Design review of the part built by this model. Coordinates are the model's own, in mm. Face numbers are marked on the shaded views. A direction names the side the tool comes from. Round coordinates to 2 decimals unless told otherwise and drop trailing zeros. Order: outer loops, then holes, each group sorted by start corner. A loop starts at its lowest first (then second) coordinate and runs counter-clockwise, first axis right, second up. Notation, with made-up numbers: (28.5, -1) - (52.5, -1) arc R19 ccw to (52.5, 30) - close; hole circle Ø5 at (65.5, -21). An arc over 180 degrees is marked (long way). Write item = value, one per line.
Autodesk Inventor part; units mm, degrees
ref_plane "XZ Plane" through (0, 0, 0) normal (0, 1, 0) x (-1, 0, 0)
sketch "Sketch1" plane through (0, 0, 0) normal (0, 1, 0) x (-1, 0, 0)
  line L0 (60.4, 85.9) -> (-60.4, 85.9)
  line L1 (-60.4, 85.9) -> (-60.4, -85.9)
  line L2 (-60.4, -85.9) -> (60.4, -85.9)
  line L3 (60.4, -85.9) -> (60.4, 85.9)
  point P0 (0, 0)
  dimension "d0" = 85.9
  dimension "d1" = 85.9
  dimension "d2" = 60.4
  dimension "d3" = 60.4
extrude "Extrusion1" add sketch "Sketch1" along normal blind 55.05
fillet "Fillet1" radius 2 6 edges at (60.4, 27.525, 85.9) (-60.4, 27.525, 85.9) (60.4, 27.525, -85.9) (-60.4, 27.525, -85.9) (60.4, 0, 0) (-60.4, 0, 0)
sketch "Sketch2" plane through (0, 55.05, 0) normal (0, 1, 0) x (1, 0, 0)
  line L0 (-58.4, -83.9) -> (58.4, -83.9)
  line L1 (58.4, -83.9) -> (58.4, 83.9)
  line L2 (58.4, 83.9) -> (-58.4, 83.9)
  line L3 (-58.4, 83.9) -> (-58.4, -83.9)
  line L4 (-60.4, 83.9) -> (-60.4, -83.9)
  line L5 (-58.4, -85.9) -> (58.4, -85.9)
  line L6 (60.4, -83.9) -> (60.4, 83.9)
  line L7 (58.4, 85.9) -> (-58.4, 85.9)
  point P0 (0, 0)
  dimension "d7" = 2
  dimension "d8" = 2
  dimension "d9" = 2
  dimension "d10" = 2
extrude "Extrusion2" cut sketch "Sketch2" against normal blind 53.05
sketch "Sketch3" plane through (0, 0, 0) normal (0, -1, 0) x (1, 0, 0)
  line L0 (-58.4, -85.9) -> (-58.4, 85.9)
  line L1 (58.4, -85.9) -> (-58.4, -85.9)
  line L2 (58.4, 85.9) -> (58.4, -85.9)
  line L3 (-58.4, 85.9) -> (58.4, 85.9)
  line L4 (-58.4, 85.9) -> (58.4, 85.9)
  line L5 (50.4, 85.9) -> (50.4, 99.9)
  line L6 (50.4, 99.9) -> (-50.4, 99.9)
  line L7 (-50.4, 99.9) -> (-50.4, 85.9)
  line L8 (-60.4, 83.9) -> (-60.4, -83.9)
  line L9 (60.4, -83.9) -> (60.4, 83.9)
  line L10 (-134.6994, 0) -> (135.5184, 0) construction
  line L11 (50.4, -85.9) -> (50.4, -99.9)
  line L12 (50.4, -99.9) -> (-50.4, -99.9)
  line L13 (-50.4, -99.9) -> (-50.4, -85.9)
  line L14 (50.4, 85.9) -> (-50.4, 85.9)
  line L15 (-50.4, -85.9) -> (50.4, -85.9)
  point P0 (0, 0)
  dimension "d13" = 10
  dimension "d14" = 10
  dimension "d15" = 14
  dimension "d16" = 0
extrude "Extrusion3" add sketch "Sketch3" against normal blind 3 contours L1 L11 L12 L13 | L7 L6 L5 L3
fillet "Fillet2" radius 4 4 edges at (-50.4, 1.5, -99.9) (50.4, 1.5, -99.9) (50.4, 1.5, 99.9) (-50.4, 1.5, 99.9)
fillet "Fillet3" radius 2 8 edges at (-59.8142, 0.5858, 85.3142) (-54.4, 0, 85.9) (59.8142, 0.5858, 85.3142) (54.4, 0, 85.9) (59.8142, 0.5858, -85.3142) (54.4, 0, -85.9) (-59.8142, 0.5858, -85.3142) (-54.4, 0, -85.9)
sketch "Sketch4" plane through (0, 2, 0) normal (0, 1, 0) x (1, 0, 0)
  circle A0 centre (-54.9, 80.4) radius 1.25
  line L0 (58.4, 85.9) -> (-58.4, 85.9)
  line L1 (-60.4, 83.9) -> (-60.4, -83.9)
  circle A1 centre (54.1, 80.4) radius 1.25
  circle A2 centre (-54.9, -79.6) radius 1.25
  circle A3 centre (54.1, -79.6) radius 1.25
  circle A4 centre (-54.9, 80.4) radius 2.25
  circle A5 centre (-54.9, -79.6) radius 2.25
  circle A6 centre (54.1, 80.4) radius 2.25
  circle A7 centre (54.1, -79.6) radius 2.25
  line L2 (-58.4, 83.9) -> (-60.4, 83.9)
  line L3 (-58.4, 83.9) -> (-58.4, 75.9)
  line L4 (-58.4, 83.9) -> (-58.4, -83.9)
  line L5 (-58.4, 85.9) -> (-58.4, 83.9)
  line L6 (-58.4, 83.9) -> (-50.4, 83.9)
  line L7 (-58.4, 83.9) -> (58.4, 83.9)
  arc A8 (-55.4407, 78.2159) -> (-58.4, 75.9) centre (-56.0141, 75.9) ccw
  arc A9 (-50.4, 83.9) -> (-52.7159, 80.9407) centre (-50.4, 81.5141) ccw
  line L8 (58.4, 83.9) -> (58.4, -83.9)
  line L9 (58.4, 83.9) -> (48.8739, 83.9)
  line L10 (58.4, 83.9) -> (58.4, 75.9)
  line L11 (58.4, -83.9) -> (58.4, 83.9)
  line L12 (58.4, -83.9) -> (-58.4, -83.9)
  line L13 (-58.4, -83.9) -> (-58.4, -75.9)
  line L14 (-58.4, -83.9) -> (-58.4, 83.9)
  line L15 (-58.4, -83.9) -> (-50.4, -83.9)
  arc A10 (-52.7997, -80.4071) -> (-50.4, -83.9) centre (-50.4, -81.3292) ccw
  arc A11 (-58.4, -75.9) -> (-55.8323, -77.5522) centre (-56.5846, -75.9) ccw
  line L16 (58.4, -83.9) -> (50.4, -83.9)
  line L17 (58.4, -83.9) -> (58.4, -75.9)
  arc A12 (55.2614, -77.6729) -> (58.4, -75.9) centre (56.33, -75.9) ccw
  arc A13 (50.4, -83.9) -> (52.1729, -80.7614) centre (50.4, -81.83) ccw
  circle A14 centre (54.5, 0) radius 1.25
  circle A15 centre (-54.5, 0) radius 1.25
  circle A16 centre (-54.5, 0) radius 2.25
  circle A17 centre (54.5, 0) radius 2.25
  line L18 (54.5, -2.25) -> (56.9, -2.25)
  line L19 (54.5, 2.25) -> (56.9, 2.25)
  line L20 (-54.5, -2.25) -> (-56.9, -2.25)
  line L21 (-54.5, 2.25) -> (-56.9, 2.25)
  line L22 (0, 85.9) -> (0, 75.9)
  line L23 (-58.4, -83.9) -> (-58.4, 83.9)
  line L24 (58.4, -83.9) -> (-58.4, -83.9)
  line L25 (-58.4, 83.9) -> (58.4, 83.9)
  arc A18 (58.4, -3.75) -> (56.9, -2.25) centre (56.9, -3.75) ccw
  line L26 (58.4, 83.9) -> (58.4, -83.9)
  arc A19 (56.9, 2.25) -> (58.4, 3.75) centre (56.9, 3.75) ccw
  arc A20 (-56.9, -2.25) -> (-58.4, -3.75) centre (-56.9, -3.75) ccw
  arc A21 (-58.4, 3.75) -> (-56.9, 2.25) centre (-56.9, 3.75) ccw
  arc A22 (51.8602, 80.6143) -> (48.8739, 83.9) centre (48.8739, 80.9) ccw
  arc A23 (58.4, 75.3135) -> (54.6571, 78.2201) centre (55.4, 75.3135) ccw
  line L27 (-58.4, 75.9) -> (-58.4, 83.7116)
  line L28 (-58.4, 75.9) -> (-58.4, 83.9)
  line L29 (-50.4, 83.9) -> (-58.4, 83.9)
  line L30 (60.4, 83.9) -> (58.4, 83.9)
  line L31 (48.8739, 83.9) -> (58.4, 83.9)
  line L32 (58.4, 83.9) -> (58.4, 75.3135)
  point P0 (0, 0)
  point P1 (58.4, -2.25)
  point P2 (58.4, 2.25)
  point P3 (-58.4, -2.25)
  point P4 (-58.4, 2.25)
  dimension "d21" = 2.5
  dimension "d23" = 5.5
  dimension "d24" = 5.5
  dimension "d27" = 109
  dimension "d30" = 160
  dimension "d33" = 4.5
  dimension "d36" = 160
  dimension "d39" = 109
  dimension "d42" = 8
  dimension "d43" = 8
  dimension "d46" = 8
  dimension "d47" = 8
  dimension "d48" = 8
  dimension "d49" = 8
  dimension "d52" = 2.5
  dimension "d53" = 2.5
  dimension "d54" = 3.9
  dimension "d56" = 3.9
  dimension "d57" = 0
  dimension "d58" = 0
  dimension "d59" = 4.5
  dimension "d60" = 4.5
  dimension "d115" = 1.5
  dimension "d116" = 1.5
  dimension "d117" = 1.5
  dimension "d118" = 1.5
  dimension "d119" = 3
  dimension "d120" = 3
sketch "Sketch6" plane through (0, 3, 0) normal (0, 1, 0) x (1, 0, 0)
  circle A0 centre (40.4, 92.9) radius 2.5
  line L0 (50.4, 85.9) -> (50.4, 95.9)
  line L1 (46.4, 99.9) -> (-46.4, 99.9)
  circle A1 centre (-39.6, 92.9) radius 2.5
  circle A2 centre (40.4, -92.1) radius 2.5
  circle A3 centre (-39.6, -92.1) radius 2.5
  circle A4 centre (0, 92.9) radius 3
  circle A5 centre (0, -92.9) radius 3
  line L2 (-50.4, -85.9) -> (50.4, -85.9)
  line L3 (0, 139.86) -> (0, -139.86)
  line L4 (50.4, 85.9) -> (-50.4, 85.9)
  point P0 (0, 0)
  dimension "d62" = 5
  dimension "d63" = 10
  dimension "d64" = 7
  dimension "d67" = 80
  dimension "d70" = 185
  dimension "d109" = 6
  dimension "d110" = 6
  dimension "d111" = 7
  dimension "d112" = 0
  dimension "d113" = 7
  dimension "d114" = 0
extrude "Extrusion5" cut sketch "Sketch6" against normal blind 3
sketch "Sketch8" plane through (0, 55.05, 0) normal (0, 1, 0) x (1, 0, 0)
  line L0 (58.4, 83.9) -> (58.4, -83.9)
  line L1 (58.4, -83.9) -> (-58.4, -83.9)
  line L2 (-58.4, -83.9) -> (-58.4, 83.9)
  line L3 (-58.4, 83.9) -> (58.4, 83.9)
  arc A0 (-60.4, -83.9) -> (-58.4, -85.9) centre (-58.4, -83.9) ccw
  line L4 (-58.4, -85.9) -> (58.4, -85.9)
  arc A1 (58.4, -85.9) -> (60.4, -83.9) centre (58.4, -83.9) ccw
  line L5 (60.4, -83.9) -> (60.4, 83.9)
  arc A2 (60.4, 83.9) -> (58.4, 85.9) centre (58.4, 83.9) ccw
  line L6 (58.4, 85.9) -> (-58.4, 85.9)
  arc A3 (-58.4, 85.9) -> (-60.4, 83.9) centre (-58.4, 83.9) ccw
  line L7 (-60.4, 83.9) -> (-60.4, -83.9)
  point P0 (0, 0)
equation "\"d7\" = d8"
equation "\"d9\" = d8"
equation "\"d10\" = d8"
properties part number "Main Enclosure Base 2"
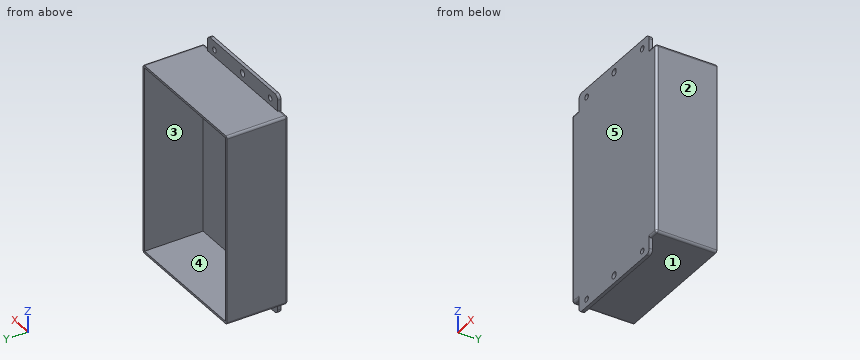
1) We need section B-B on y = 27. Write out the cut boundary in (x, z).
Findings:
outline = (-60.4, -83.9) arc R2 ccw to (-58.4, -85.9) - (58.4, -85.9) arc R2 ccw to (60.4, -83.9) - (60.4, 83.9) arc R2 ccw to (58.4, 85.9) - (-58.4, 85.9) arc R2 ccw to (-60.4, 83.9) - close; hole (-58.4, -83.9) - (58.4, -83.9) - (58.4, 83.9) - (-58.4, 83.9) - close
2) For the marked faces 4 and 5, list the 3-axis set-ups (+Z, -Z, +X, -X, +Y, -Y) from which the entire face can be reached by the end or side of a thin tool; tool diameter is ignored.
Findings:
face_4 = +Y
face_5 = +Z, -Z, +X, -X, -Y
3) The part is to be moulded in two halves that separate along X. For the marked faces 1, 2 and 3, say which applies: released by +X, released by -X, zero draft, split by the parting line, or undercut.
Findings:
face_1 = zero draft
face_2 = released by +X
face_3 = undercut
4) We need section D-D on x = -27. Write out the cut boundary in (y, z), and give its area (3 significant figures).
Findings:
outline = (0, -99.9) - (3, -99.9) - (3, -85.9) - (55.05, -85.9) - (55.05, -83.9) - (2, -83.9) - (2, 83.9) - (55.05, 83.9) - (55.05, 85.9) - (3, 85.9) - (3, 99.9) - (0, 99.9) - close
area = 640 mm^2
5) Clearance check with flat-ended pins moving along their axes: pin 1 Ø8 at (x, z) = (0, -92.9) entering from +Y; pin 2 Ø12 at (x, y) = (48, 22.5) entering from +Z; pin 3 Ø6 at (x, z) = (-19, 2.5) entering from +Y; pin 4 Ø3.5 at (x, z) = (0, 92.9) entering from +Y. State where each tip first meets the part, or that it passes through.
Findings:
pin_1 = 3
pin_2 = 85.9
pin_3 = 2
pin_4 = through
6) We need section C-C on z = 39.5. Write out the cut boundary in (x, y).
Findings:
outline = (-60.4, 2) arc R2 ccw to (-58.4, 0) - (58.4, 0) arc R2 ccw to (60.4, 2) - (60.4, 55.05) - (58.4, 55.05) - (58.4, 2) - (-58.4, 2) - (-58.4, 55.05) - (-60.4, 55.05) - close
7) We need section A-A on x = 40.4. Write out the cut boundary in (y, z), and give its area (3 significant figures).
Findings:
outline = (0, -99.9) - (3, -99.9) - (3, -95.4) - (0, -95.4) - close; (0, -90.4) - (3, -90.4) - (3, -85.9) - (55.05, -85.9) - (55.05, -83.9) - (2, -83.9) - (2, 83.9) - (55.05, 83.9) - (55.05, 85.9) - (3, 85.9) - (3, 89.6) - (0, 89.6) - close; (0, 94.6) - (3, 94.6) - (3, 99.9) - (0, 99.9) - close
area = 610 mm^2
8) To check wall thickness, follow L1, parallel to Z at x = 40.4, y = 1.25; L2, parallel to Z at x = 0, y = 1; L3, parallel to X at y = 1.85, z = -92.9. State the ranges of each line that lie inside material, in increasing order. Write a range as from..to.
Findings:
L1 = -99.9..-95.4, -90.4..89.6, 94.6..99.9
L2 = -99.9..-95.9, -89.9..89.9, 95.9..99.9
L3 = -50.4..-42.1, -37.1..-3, 3..37.9, 42.9..50.4
